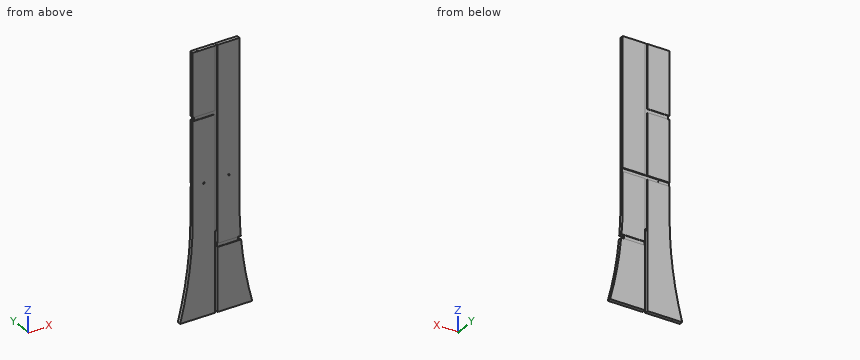
```python
from build123d import *

# Parameters (mm, degrees)
F1_DEPTH       = 12.7
F28_W          = 19.05
F28_H          = 558.8
F29_DEPTH      = 25.4
F3_D           = 3.175
F3_DEPTH       = 63.5
F3_CBORE_D     = 12.7
F3_CBORE_DEPTH = 6.35
F3_TIP         = 0.9538662327
F5_D           = 3.175
F5_DEPTH       = 63.5
F5_TIP         = 0.9538662327
F7_D           = 3.175
F7_DEPTH       = 63.5
F7_TIP         = 0.9538662327
F8_W           = 330.2
F8_H           = 25.4
F9_DEPTH       = 6.35
F10_W          = 19.05
F10_H          = 1270
F11_DEPTH      = 3.175
F12_W          = 19.05
F12_H          = 342.9
F13_DEPTH      = 3.175
F14_W          = 19.05
F14_H          = 901.7
F15_DEPTH      = 3.175
F17_W          = 50.8
F17_H          = 25.4
F18_DEPTH      = 25.4
F16_W          = 193.68262
F16_H          = 12.7
F19_DEPTH      = 3.175
F20_W          = 203.2
F20_H          = 25.4
F21_DEPTH      = 3.175
F22_W          = 19.05
F22_H          = 25.4
F23_DEPTH      = 25.4
F24_W          = 158.75
F24_H          = 25.4
F25_DEPTH      = 3.175
F26_W          = 158.75
F26_H          = 25.4
F27_DEPTH      = 3.175


with BuildPart() as f1:
    # F0 (on Front) → F1 (new body, symmetric)
    with BuildSketch(Plane.XZ):
        with BuildLine():
            Line((165.1, 1828.8), (0, 1828.8))
            Line((0, 1828.8), (-165.1, 1828.8))
            Line((-165.1, 1828.8), (-165.1, 685.8))
            ThreePointArc((-165.1, 685.8), (-187.4175900274, 340.0309838924), (-254, 0))
            Line((-254, 0), (0, 0))
            Line((0, 0), (254, 0))
            ThreePointArc((254, 0), (187.4175900273, 340.0309838924), (165.1, 685.8))
            Line((165.1, 685.8), (165.1, 1828.8))
        make_face()
    extrude(amount=F1_DEPTH, both=True)

    # F28 (on face) → F29 (cut)
    with BuildSketch(Plane.XZ.offset(12.7)):
        with Locations((0, 279.4)):
            Rectangle(F28_W, F28_H)
    extrude(amount=-F29_DEPTH, mode=Mode.SUBTRACT)

    # F3
    with Locations(Plane.XZ.offset(12.7)):
        with Locations((-88.9, 914.4), (88.9, 914.4)):
            CounterBoreHole(F3_D / 2, F3_CBORE_D / 2, F3_CBORE_DEPTH, depth=F3_DEPTH)
            with Locations((0, 0, -(F3_DEPTH + F3_TIP / 2))):  # 118° drill point
                Cone(0, F3_D / 2, F3_TIP, mode=Mode.SUBTRACT)

    # F5
    with Locations(Plane.XY.offset(1828.8)):
        with Locations((-127, 0), (127, 0)):
            Hole(F5_D / 2, depth=F5_DEPTH)
            with Locations((0, 0, -(F5_DEPTH + F5_TIP / 2))):  # 118° drill point
                Cone(0, F5_D / 2, F5_TIP, mode=Mode.SUBTRACT)

    # F7
    with Locations(Plane(origin=(0, 0, 0), x_dir=(1, 0, 0), z_dir=(0, 0, -1))):
        with Locations((-190.5, 0), (190.5, 0)):
            Hole(F7_D / 2, depth=F7_DEPTH)
            with Locations((0, 0, -(F7_DEPTH + F7_TIP / 2))):  # 118° drill point
                Cone(0, F7_D / 2, F7_TIP, mode=Mode.SUBTRACT)

    # F8 (on face) → F9 (cut)
    with BuildSketch(Plane(origin=(0, 12.7, 0), x_dir=(-1, 0, 0), z_dir=(0, 1, 0))):
        with Locations((0, 914.4)):
            Rectangle(F8_W, F8_H)
    extrude(amount=-F9_DEPTH, mode=Mode.SUBTRACT)

    # F10 (on face) → F11 (cut)
    with BuildSketch(Plane.XZ.offset(12.7)):
        with Locations((0, 1193.8)):
            Rectangle(F10_W, F10_H)
    extrude(amount=-F11_DEPTH, mode=Mode.SUBTRACT)

    # F12 (on face) → F13 (cut)
    with BuildSketch(Plane(origin=(0, 12.7, 0), x_dir=(-1, 0, 0), z_dir=(0, 1, 0))):
        with Locations((0, 730.25)):
            Rectangle(F12_W, F12_H)
    extrude(amount=-F13_DEPTH, mode=Mode.SUBTRACT)

    # F14 (on face) → F15 (cut)
    with BuildSketch(Plane(origin=(0, 12.7, 0), x_dir=(-1, 0, 0), z_dir=(0, 1, 0))):
        with Locations((0, 1377.95)):
            Rectangle(F14_W, F14_H)
    extrude(amount=-F15_DEPTH, mode=Mode.SUBTRACT)

    # F17 (on face) → F18 (cut)
    with BuildSketch(Plane.XZ.offset(12.7)):
        with Locations((180.975, 457.2)):
            Rectangle(F17_W, F17_H)
    extrude(amount=-F18_DEPTH, mode=Mode.SUBTRACT)

    # F16 (on face) → F19 (cut)
    with BuildSketch(Plane.XZ.offset(12.7)):
        with Locations((96.84131, 463.55)):
            Rectangle(F16_W, F16_H)
        with Locations((96.84131, 450.85)):
            Rectangle(F16_W, F16_H)
    extrude(amount=-F19_DEPTH, mode=Mode.SUBTRACT)

    # F20 (on face) → F21 (cut)
    with BuildSketch(Plane(origin=(0, 12.7, 0), x_dir=(-1, 0, 0), z_dir=(0, 1, 0))):
        with Locations((-101.6, 457.2)):
            Rectangle(F20_W, F20_H)
    extrude(amount=-F21_DEPTH, mode=Mode.SUBTRACT)

    # F22 (on face) → F23 (cut)
    with BuildSketch(Plane.XZ.offset(12.7)):
        with Locations((-165.1, 1371.6)):
            Rectangle(F22_W, F22_H)
    extrude(amount=-F23_DEPTH, mode=Mode.SUBTRACT)

    # F24 (on face) → F25 (cut)
    with BuildSketch(Plane.XZ.offset(12.7)):
        with Locations((-85.725, 1371.6)):
            Rectangle(F24_W, F24_H)
    extrude(amount=-F25_DEPTH, mode=Mode.SUBTRACT)

    # F26 (on face) → F27 (cut)
    with BuildSketch(Plane(origin=(0, 12.7, 0), x_dir=(-1, 0, 0), z_dir=(0, 1, 0))):
        with Locations((85.725, 1371.6)):
            Rectangle(F26_W, F26_H)
    extrude(amount=-F27_DEPTH, mode=Mode.SUBTRACT)


solid = f1.part
```
The listing builds one solid part. Answer for the finished solid, in the listing's coordinates (mm). Round coordinates to 2 decimals unless told otherwise and drop trailing zeros. Loops run counter-clockwise (first coordinate to the right, second up) from the corner with the lowest first, then second, coordinate; pieces in that order, holes last.
Q1. Section B-B, the plane z = 253 is taken. Determine the outline of the cut face in (x, y) (3 decimals), then the cut area to 3 significant figures.
Q2. Find the intervals of material crossed by line 1 (Z direction, x = 163, y = 7.75); line 2 (X direction, y = 0, z = 1813); line 3 (Z direction, x = 88.9, y = -11), in increasing order.
Q3. Section A-A, the plane z = 793.5 is taken. Determine the outline of the cut face in (x, y) (3 decimals).
Q4. Given pin 1 Ø9.5 at (y, z) = (3.5, 459) entering from +X (3 decimals); pin 2 Ø1 at (y, z) = (3.5, 713) entering from -X; pin 3 Ø5 at (x, z) = (-88.9, 914.4) entering from +Y; pin 4 Ø4 at (x, y) = (-127, 0) entering from +Z, each flat-ended and moving along its own axis, determine where each tip first touches the part or whether it passes through.
Completed:
1. outline: (-200.15, -12.7) - (-9.525, -12.7) - (-9.525, 12.7) - (-200.15, 12.7) - close; (9.525, -12.7) - (200.15, -12.7) - (200.15, 12.7) - (9.525, 12.7) - close
1. area: 9,680 mm2
2. line 1: z = 0 to 444.5, 469.9 to 901.7, 927.1 to 1828.8
2. line 2: x = -165.1 to -128.59, -125.41 to 125.41, 128.59 to 165.1
2. line 3: z = 0 to 444.5, 469.9 to 908.05, 920.75 to 1828.8
3. outline: (-165.1, -12.7) - (-9.525, -12.7) - (-9.525, -9.525) - (9.525, -9.525) - (9.525, -12.7) - (165.1, -12.7) - (165.1, 12.7) - (9.525, 12.7) - (9.525, 9.525) - (-9.525, 9.525) - (-9.525, 12.7) - (-165.1, 12.7) - close
4. pin 1: stops at x = 155.575
4. pin 2: stops at x = -165.1
4. pin 3: stops at y = 6.35
4. pin 4: stops at z = 1828.8
